Check sheet for the modelled part. Datum: model origin and axes. Units: mm. Face numbers are marked on the shaded views. A direction names the side the tool comes from. Round coordinates to 2 decimals unless told otherwise and drop trailing zeros. Loops run counter-clockwise (first coordinate to the right, second up) from the corner with the lowest first, then second, coordinate; pieces in that order, holes last. Notation, with made-up numbers: (-26.75, 12) - (-18.75, 12) arc R21 cw to (-18.75, 38) - close; hole circle Ø11 at (-31.5, -40). An arc over 180 degrees is marked (long way). Put each result on its own line as item: value. Start each with the question number.
Item 1: Section check C-C, the plane z = 15.25. Record the cut outline in (x, y), and give its area (3 significant figures).
Item 2: Draft check along Y on the marked faces 1, 2 and 3. Enter one of: pulls with the +Y half, pulls with the -Y half, needs draft (parallel to the pull), parting line crosses it, or undercut.
Item 3: Material ranges on line 1 along Y through (x, z) = (0, 9.75); line 2 along X through (y, z) = (-9, 25.25); line 3 along Y through (x, z) = (-29, 24.75), recorded low to high.
Item 4: Gauge pin test, flat ends, axial feed: pin 1 Ø7 at (x, z) = (-31, 2) entering from +Y; pin 2 Ø5 at (x, z) = (28, 3) entering from +Y; pin 3 Ø6.5 at (x, y) = (27.5, 0) entering from -Z. Record the tip position at first contact, or that the pin passes through.
Item 5: Tool access check on the marked faces 4, 5 and 6. Record the directions out of +Z, -Z, +X, -X, +Y, -Y that give a thin tool (end or side, any length) a straight path to the whole face; none if there is none.
Item 6: Section check D-D, the plane x = 14.5. Record the cut outline in (y, z), and give its area (3 significant figures).
Item 7: Section check B-B, the plane z = 22. Record the cut outline in (x, y), and give its area (3 significant figures).
Item 8: Section check A-A, the plane y = 0. Record the cut outline in (x, z), and give its area (3 significant figures).
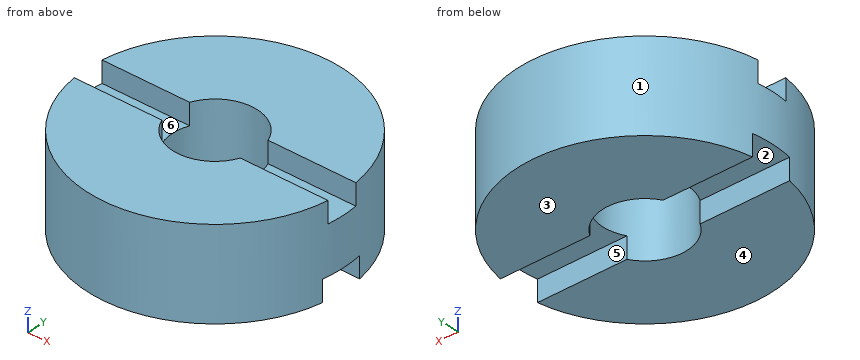
from build123d import *

# Parameters (mm, degrees)
F0_R     = 38.1
F0_R_2   = 12.6238
F1_DEPTH = 26.924
F3_DEPTH = 6.35
F5_DEPTH = 6.35


with BuildPart() as f1:
    # F0 (on Top) → F1 (new body)
    with BuildSketch(Plane.XY):
        Circle(F0_R)
        Circle(F0_R_2, mode=Mode.SUBTRACT)
    extrude(amount=F1_DEPTH)

    # F2 (on face) → F3 (cut)
    with BuildSketch(Plane.XY.offset(26.924)):
        with BuildLine():
            Line((-11.6909760153, 4.7625), (-37.8011718568, 4.7625))
            ThreePointArc((-37.8011718568, 4.7625), (-38.0252195769, 2.3859329679), (-38.1, 0))
            ThreePointArc((-38.1, 0), (-38.0252195769, -2.3859329679), (-37.8011718568, -4.7625))
            Line((-37.8011718568, -4.7625), (-11.6909760153, -4.7625))
            ThreePointArc((-11.6909760153, -4.7625), (-12.6238, 0), (-11.6909760153, 4.7625))
        make_face()
        with BuildLine():
            ThreePointArc((38.1, 0), (38.0252195769, 2.3859329679), (37.8011718568, 4.7625))
            Line((37.8011718568, 4.7625), (11.6909760153, 4.7625))
            ThreePointArc((11.6909760153, 4.7625), (12.3883991997, 2.426497828), (12.6238, 0))
            ThreePointArc((12.6238, 0), (12.3883991997, -2.426497828), (11.6909760153, -4.7625))
            Line((11.6909760153, -4.7625), (37.8011718568, -4.7625))
            ThreePointArc((37.8011718568, -4.7625), (38.0252195769, -2.3859329679), (38.1, 0))
        make_face()
    extrude(amount=-F3_DEPTH, mode=Mode.SUBTRACT)

    # F4 (on face) → F5 (cut)
    with BuildSketch(Plane(origin=(0, 0, 0), x_dir=(1, 0, 0), z_dir=(0, 0, -1))):
        with BuildLine():
            Line((-10.9104457489, 6.35), (-37.5671066227, 6.35))
            ThreePointArc((-37.5671066227, 6.35), (-37.9665429182, 3.1861605167), (-38.1, 0))
            ThreePointArc((-38.1, 0), (-37.9665429182, -3.1861605167), (-37.5671066227, -6.35))
            Line((-37.5671066227, -6.35), (-10.9104457489, -6.35))
            ThreePointArc((-10.9104457489, -6.35), (-12.6238, 0), (-10.9104457489, 6.35))
        make_face()
        with BuildLine():
            ThreePointArc((38.1, 0), (37.9665429182, 3.1861605167), (37.5671066227, 6.35))
            Line((37.5671066227, 6.35), (10.9104457489, 6.35))
            ThreePointArc((10.9104457489, 6.35), (12.1879368944, 3.2885438567), (12.6238, 0))
            ThreePointArc((12.6238, 0), (12.1879368944, -3.2885438567), (10.9104457489, -6.35))
            Line((10.9104457489, -6.35), (37.5671066227, -6.35))
            ThreePointArc((37.5671066227, -6.35), (37.9665429182, -3.1861605167), (38.1, 0))
        make_face()
    extrude(amount=-F5_DEPTH, mode=Mode.SUBTRACT)


solid = f1.part
Check result:
1. outline: circle Ø76.2 at (0, 0); hole circle Ø25.25 at (0, 0)
1. area: 4,060 mm²
2. face 1: parting line crosses it
2. face 2: undercut
2. face 3: needs draft
3. line 1: -38.1 to -12.62, 12.62 to 38.1
3. line 2: -37.02 to -8.85, 8.85 to 37.02
3. line 3: -24.71 to -4.76, 4.76 to 24.71
4. pin 1: y = 26.37
4. pin 2: y = 28.31
4. pin 3: z = 6.35
5. face 4: -Z, +X, -X, +Y, -Y
5. face 5: -Z, +X, -X
5. face 6: +Z, +X, -X
6. outline: (-35.23, 0) - (-6.35, 0) - (-6.35, 6.35) - (6.35, 6.35) - (6.35, 0) - (35.23, 0) - (35.23, 26.92) - (4.76, 26.92) - (4.76, 20.57) - (-4.76, 20.57) - (-4.76, 26.92) - (-35.23, 26.92) - close
6. area: 1,760 mm²
7. outline: (-37.8, -4.76) arc R38.1 ccw to (37.8, -4.76) - (11.69, -4.76) arc R12.62 cw to (-11.69, -4.76) - close; (-37.8, 4.76) - (-11.69, 4.76) arc R12.62 cw to (11.69, 4.76) - (37.8, 4.76) arc R38.1 ccw to start
7. area: 3,570 mm²
8. outline: (-38.1, 6.35) - (-12.62, 6.35) - (-12.62, 20.57) - (-38.1, 20.57) - close; (12.62, 6.35) - (38.1, 6.35) - (38.1, 20.57) - (12.62, 20.57) - close
8. area: 725 mm²
